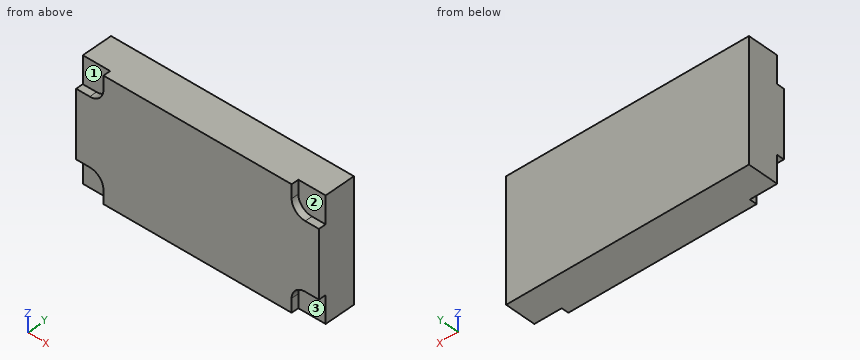
```python
from build123d import *

# Parameters (mm, degrees)
CROQUIS_BASE_W          = 40
CROQUIS_BASE_H          = 20
SALIENTE_EXTRUIR1_DEPTH = 6.25
CORTAR_EXTRUIR1_DEPTH   = 1.2


with BuildPart() as part:
    # Croquis base → Saliente-Extruir1 (new body)
    with BuildSketch(Plane(origin=(0, 0, 0), x_dir=(1, 0, 0), z_dir=(0, 1, 0))):
        Rectangle(CROQUIS_BASE_W, CROQUIS_BASE_H)
    extrude(amount=SALIENTE_EXTRUIR1_DEPTH)

    # Croquis base detalles → Cortar-Extruir1 (cut)
    with BuildSketch(Plane.XZ):
        with BuildLine():
            Line((15.5, 10), (15.5, 7.75))
            ThreePointArc((15.5, 7.75), (16.159009742, 6.159009742), (17.75, 5.5))
            Line((17.75, 5.5), (20, 5.5))
            Line((20, 5.5), (20, 10))
            Line((20, 10), (15.5, 10))
        make_face()
        with BuildLine():
            Line((-20, 10), (-15.5, 10))
            Line((-15.5, 10), (-15.5, 7.75))
            ThreePointArc((-15.5, 7.75), (-16.159009742, 6.159009742), (-17.75, 5.5))
            Line((-17.75, 5.5), (-20, 5.5))
            Line((-20, 5.5), (-20, 10))
        make_face()
        with BuildLine():
            Line((20, -10), (15.5, -10))
            Line((15.5, -10), (15.5, -7.75))
            ThreePointArc((15.5, -7.75), (16.159009742, -6.159009742), (17.75, -5.5))
            Line((17.75, -5.5), (20, -5.5))
            Line((20, -5.5), (20, -10))
        make_face()
        with BuildLine():
            Line((-15.5, -10), (-15.5, -7.75))
            ThreePointArc((-15.5, -7.75), (-16.159009742, -6.159009742), (-17.75, -5.5))
            Line((-17.75, -5.5), (-20, -5.5))
            Line((-20, -5.5), (-20, -10))
            Line((-20, -10), (-15.5, -10))
        make_face()
    extrude(amount=-CORTAR_EXTRUIR1_DEPTH, mode=Mode.SUBTRACT)


solid = part.part
```
Geometry: final body of the model. Coordinates: model frame, mm. Face numbers are marked on the shaded views. A direction names the side the tool comes from. Give positions to 0.01 mm unless a question says otherwise; leave off trailing zeros. Loops run counter-clockwise (first coordinate to the right, second up) from the corner with the lowest first, then second, coordinate; pieces in that order, holes last. Notation, with made-up numbers: (19, 57.25) -> (39, 57.25) arc R24 ccw to (39, 89.25) -> close; hole circle Ø6 at (6, -27). An arc over 180 degrees is marked (long way). Use one line per item in the form item = value.
Item 1: Line query: probe 1 along X at (y, z) = (0.5, 8.75); probe 2 along Z at (x, y) = (-16, 0.75). Output: solid intervals per line, ascending.
A:
probe_1 = -15.5 to 15.5
probe_2 = -6.34 to 6.34
Item 2: Section query A-A on z = -8.25. Output: boundary loops of the cut face in (x, y).
A:
outline = (-20, 1.2) -> (-15.5, 1.2) -> (-15.5, 0) -> (15.5, 0) -> (15.5, 1.2) -> (20, 1.2) -> (20, 6.25) -> (-20, 6.25) -> close
Item 3: Access query for the marked faces 1, 2 and 3. Directions: +Z, -Z, +X, -X, +Y, -Y. A direction counts if a zero-diameter tool reaches every point of the face in a straight line with its end or side. Return the directions, or none.
A:
face_1 = +Z, -X, -Y
face_2 = +Z, +X, -Y
face_3 = -Z, +X, -Y
Item 4: Pin query (flat end, axial travel): P1, Ø1.3, axis at x = -18.5, y = 0.5, coming from the +Z side; P2, Ø1, axis at x = 18.5, y = 1, coming from the -Z side; P3, Ø0.6, axis at y = 0.5, z = 9, coming from the +X side; P4, Ø1.3, axis at x = -18, z = 9, coming from the -Y side. Return the tip coordinate at first contact, or that it passes through.
A:
P1 = 5.5
P2 = -10
P3 = 15.5
P4 = 1.2
Item 5: Section query B-B on x = 16.5. Output: boundary loops of the cut face in (y, z).
A:
outline = (0, -5.88) -> (1.2, -5.88) -> (1.2, -10) -> (6.25, -10) -> (6.25, 10) -> (1.2, 10) -> (1.2, 5.88) -> (0, 5.88) -> close
